The drawing under review shows one solid part. Ordinate dimensions are in mm from its lowest x, y, z. Coordinates: 2 decimals unless noted, no trailing zeros. Loops run counter-clockwise (first coordinate to the right, second up) from the corner with the lowest first, then second, coordinate; pieces in that order, holes last. Notation, with made-up numbers: M 88.25,45.25 L 102.25,45.25 A6 cw 102.25,51.25 Z; hole C -40,74 d7. An arc over 180 degrees is marked long. Use one line per item in the form item = value.
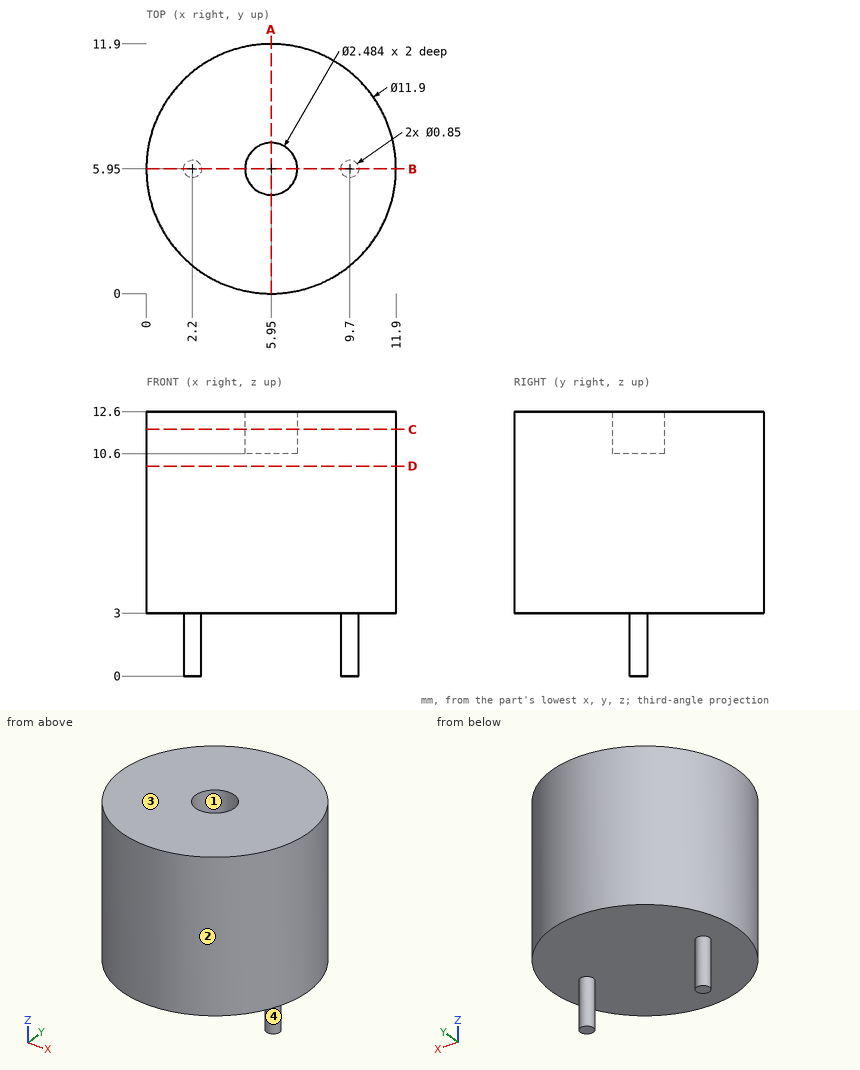
1. Draft analysis for pull direction X (two halves, no side actions). For the marked faces 1, 2, 3 and 4, state which applies: +X half, -X half, draft (parallel to the pull), parting line (faces both ways), or undercut.
Computed values:
face_1 = undercut
face_2 = parting line
face_3 = draft
face_4 = undercut
2. Wall thickness on line 1 along Y through (x, z) = (5.95, 11.45); line 2 along Z through (x, y) = (6.5, 6.5); line 3 along Z through (x, y) = (8.5, 10.25): over which ranges is each line inside the solid? List them lowest first. Write a range as from..to.
Computed values:
line_1 = 0..4.71, 7.19..11.9
line_2 = 3..10.6
line_3 = 3..12.6
3. Consider section C-C on z = 11.75. Write out the cut boundary in (x, y).
Computed values:
outline = C 5.95,5.95 d11.9; hole C 5.95,5.95 d2.48
4. Consider section B-B on y = 5.95. Write out the cut boundary in (x, z) (3 decimals).
Computed values:
outline = M 0,3 L 1.775,3 L 1.775,0 L 2.625,0 L 2.625,3 L 9.275,3 L 9.275,0 L 10.125,0 L 10.125,3 L 11.9,3 L 11.9,12.6 L 7.192,12.6 L 7.192,10.6 L 4.708,10.6 L 4.708,12.6 L 0,12.6 Z
5. Consider section A-A on x = 5.95. Write out the cut boundary in (y, z).
Computed values:
outline = M 0,3 L 11.9,3 L 11.9,12.6 L 7.19,12.6 L 7.19,10.6 L 4.71,10.6 L 4.71,12.6 L 0,12.6 Z
6. Consider section D-D on z = 10. Write out the cut boundary in (x, y).
Computed values:
outline = C 5.95,5.95 d11.9
7. For pin 1 Ø2 at (x, y) = (4.5, 7) entering from -Z; pin 2 Ø2 at (x, z) = (4.5, 10.5) entering from +Y; pin 3 Ø1.2 at (x, y) = (6.5, 6) entering from +Z, all flat-tipped, find the tip position at first contact; note any pin that passes through.
Computed values:
pin_1 = 3
pin_2 = 11.88
pin_3 = 10.6
